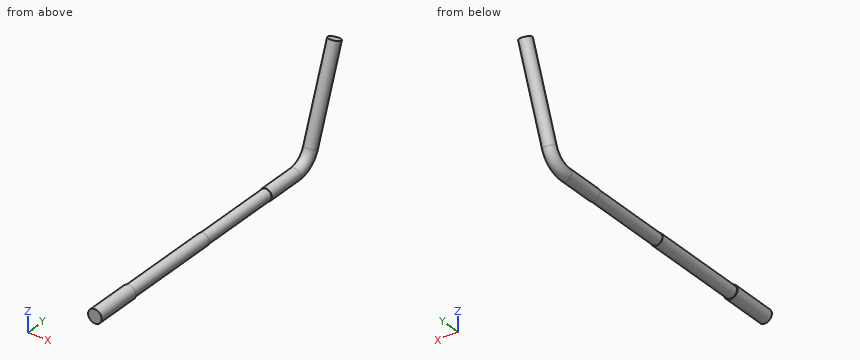
from build123d import *

# Parameters (mm, degrees)
SKETCH2_R         = 0.8
SKETCH4_R         = 0.9
EXTRUDE1_DEPTH    = 6
SKETCH5_OUTSIDE_W = 12.85
SKETCH5_OUTSIDE_H = 25.724
SKETCH5_OUTSIDE_R = 0.75
EXTRUDE3_DEPTH    = 11


with BuildPart() as part:
    # Sweep1: sweep along a path in Sketch1
    with BuildLine(Plane(origin=(0, 0, 0), x_dir=(0, 0, -1), z_dir=(1, 0, 0))) as sweep1_path:
        Line((4.5, 0), (4.5, 35))
        ThreePointArc((4.5, 35), (3.957456133, 36.720729309), (2.52606043, 37.819077862))
        Line((2.52606043, 37.819077862), (-9, 42.014220777))
    # Sketch2 → Sweep1 (sweep)
    with BuildSketch(Plane(origin=(0, 0, 0), x_dir=(1, 0, 0), z_dir=(0, 1, 0))):
        with Locations((0, 4.5)):
            Circle(SKETCH2_R)
    sweep(path=sweep1_path.line)

    # Sketch4 → Extrude1 (add)
    with BuildSketch(Plane(origin=(0, 0, 0), x_dir=(1, 0, 0), z_dir=(0, 1, 0))):
        with Locations((0, 4.5)):
            Circle(SKETCH4_R)
    extrude(amount=EXTRUDE1_DEPTH)

    # Sketch5 outside → Extrude3 (cut)
    with BuildSketch(Plane(origin=(0, 19, 0), x_dir=(-1, 0, 0), z_dir=(0, 1, 0))):
        with Locations((0, 1.937)):
            Rectangle(SKETCH5_OUTSIDE_W, SKETCH5_OUTSIDE_H)
        with Locations((0, -4.5)):
            Circle(SKETCH5_OUTSIDE_R, mode=Mode.SUBTRACT)
    extrude(amount=EXTRUDE3_DEPTH, mode=Mode.SUBTRACT)


solid = part.part
Input: part model. Units: mm. Frame: model coordinates. Give positions to 0.01 mm unless a question says otherwise; leave off trailing zeros. Order: outer loops, then holes, each group sorted by start corner. A loop starts at its lowest first (then second) coordinate and runs counter-clockwise, first axis right, second up. Notation, with made-up numbers: (46.25, 2) -> (64.25, 2) arc R26 cw to (64.25, 23) -> close; hole circle Ø7 at (34, -26). An arc over 180 degrees is marked (long way). Use one line per item in the form item = value.
1) Line query: probe 1 along Z at (x, y) = (0, 20); probe 2 along Z at (x, y) = (0, 14); probe 3 along Y at (x, z) = (-0.15, 1). Output: solid intervals per line, ascending.
Response values:
probe_1 = -5.25 to -3.75
probe_2 = -5.3 to -3.7
probe_3 = 38.27 to 39.94
2) First-contact query: pin 1 Ø0.5 at (x, z) = (-0.5, -4.5) entering from +Y; pin 2 Ø5 at (y, z) = (13.5, -2) entering from -X; pin 3 Ø1 at (x, z) = (-0.5, -3) entering from +Y; pin 4 Ø2 at (y, z) = (24.5, -1) entering from -X. Flat tips, straight axial feed; report the tip coordinate or a pass-through.
Response values:
pin_1 = 37.45
pin_2 = -0.8
pin_3 = 38.62
pin_4 = through
3) Section B-B, the plane y = 26. Return loops of the section in (x, z).
Response values:
outline = circle Ø1.5 at (0, -4.5)
4) Section C-C, the plane y = 9. Return loops of the section in (x, z).
Response values:
outline = circle Ø1.6 at (0, -4.5)
5) Section A-A, the plane x = 0. Return loops of the section in (y, z).
Response values:
outline = (0, -5.4) -> (6, -5.4) -> (6, -5.3) -> (19, -5.3) -> (19, -5.25) -> (30, -5.25) -> (30, -5.3) -> (35, -5.3) arc R3.8 ccw to (38.57, -2.8) -> (42.77, 8.73) -> (41.26, 9.27) -> (37.07, -2.25) arc R2.2 cw to (35, -3.7) -> (30, -3.7) -> (30, -3.75) -> (19, -3.75) -> (19, -3.7) -> (6, -3.7) -> (6, -3.6) -> (0, -3.6) -> close
